Could you check a few things on this model? Use its own coordinates, in mm. A direction names the side the tool comes from. Give positions to 0.01 mm unless a question says otherwise; leave off trailing zeros. Write each loop counter-clockwise with the first axis right and the second up, starting at its lowest first coordinate (ties: lowest second). Pieces come first, ordered by that corner, then holes. Notation, with made-up numbers: (6, 13) - (18, 13) arc R21 ccw to (18, 28) - close; hole circle Ø10 at (64.5, -6.5). An arc over 180 degrees is marked (long way). Answer as CSV lines item,"result". Start each with the question number.
Q1. If I drill on line 1 along Y through (x, z) = (-18.5, 11.75); line 2 along X through (y, z) = (7.5, 13); line 3 along Y through (x, z) = (-8.5, 17.5), over which ranges is the centre line in solid material (lowest first)?
Q2. On a 3-axis mill with a long thin cutter (end or side, diameter ignored), from which of +Z, -Z, +X, -X, +Y, -Y can I reach the whole of each face in a straight line? I mean faces 4 (the face through (-10.747, -2.869, 19.184)), 5 (the face through (-8.482, -2.9, 5.6)), 6 (the face through (10, 1.232, 11)), 7 (the face through (-1.1, 3.432, 1.8)). Say none if no direction works.
Q3. We'd pull the mould along X, two halves only. Please class faces 1 (the face through (-22, -3, 8)), 2 (the face through (-19.86, 7.25, 17.38)), 3 (the face through (10, 5, 13.9)): pulls with the +X half, pulls with the -X half, needs draft (parallel to the pull), parting line crosses it, or undercut.
Q4. Imagine slicing it at D-D on z = 3.5. List the corners of the cut face in (x, y) for me.
Q5. Imagine slicing it at B-B on z = 8.75. List the corners of the cut face in (x, y) for me.
Q6. Imagine slicing it at A-A on y = 2. List the corners of the cut face in (x, z) for me, and give its area (3 significant figures).
Q7. Imagine slicing it at C-C on x = -18. List the corners of the cut face in (y, z) for me.
Q8. Will these pins go through, and if not, where does the flat tip stop? pin 1 Ø1.5 at (x, z) = (-0.5, 10) entering from +Y; pin 2 Ø8 at (y, z) = (0, 10) entering from -X; pin 3 Ø1 at (y, z) = (-2, 16.5) entering from -X; pin 4 Ø1.4 at (x, z) = (10, 12) entering from +Y.
```python
from build123d import *

# Parameters (mm, degrees)
F0_W          = 26
F0_H          = 22
F1_DEPTH      = 22
F2_R          = 9
F3_DEPTH      = 20
F4_W          = 15
F4_H          = 12.4
F5_DEPTH      = 22.001
F6_W          = 22
F6_H          = 22
F7_DEPTH      = 14
F8_W          = 18.7
F8_H          = 6
F9_DEPTH      = 12
F10_R         = 1.778
F11_DEPTH     = 40.001
F12_SIZE      = 1.5
F13_SIZE2     = 7.1236589649
F13_SIZE      = 16
F13_2_SIZE2   = 7.1236589649
F13_2_SIZE    = 16
F14_T1_DEPTH  = 27.800912408
F14_T3_DEPTH  = 27.800912408
F15_W         = 2.8
F15_H         = 5.8
F16_DEPTH     = 7
F17_W         = 22
F17_H         = 22
F18_DEPTH     = 1
F19_R         = 3.048
F20_DEPTH     = 26.5
F21_R         = 1.778
F22_DEPTH     = 6
F23_T1_DEPTH  = 2.5403411844
F23_T3_DEPTH  = 2.5403411844
F23_T5_DEPTH  = 2.5403411844
F23_T7_DEPTH  = 2.5403411844
F23_T9_DEPTH  = 32.2867319519
F23_T11_DEPTH = 32.2867319519
F23_T13_DEPTH = 30.3695452806
F24_T4_DEPTH  = 41.5282991577
F24_T10_DEPTH = 41.5282991577
F24_T16_DEPTH = 41.5282991577
F24_T22_DEPTH = 41.5282991577
F24_T28_DEPTH = 41.5282991577
F24_T34_DEPTH = 41.5282991577
F24_T40_DEPTH = 41.5282991577
F24_T46_DEPTH = 41.5282991577


# Not quite as in the source:
# - a fillet or chamfer that OpenCascade refuses, or shapes differently, is made with other operations: its cross-section is extruded or revolved along the edge and cut away or added


with BuildPart() as f1:
    # F0 (on Top) → F1 (new body)
    with BuildSketch(Plane.XY):
        with Locations((-0.9824799188, -2.7680952549)):
            Rectangle(F0_W, F0_H)
    extrude(amount=F1_DEPTH)

    # F2 (on face) → F3 (cut)
    with BuildSketch(Plane(origin=(0, 8.2319047451, 0), x_dir=(-1, 0, 0), z_dir=(0, 1, 0))):
        with Locations((0.9824799188, 11)):
            Circle(F2_R)
    extrude(amount=-F3_DEPTH, mode=Mode.SUBTRACT)

    # F4 (on face) → F5 (cut, through all)
    with BuildSketch(Plane.XY.offset(22)):
        with Locations((-0.9824799188, -2.7680952549)):
            Rectangle(F4_W, F4_H)
    extrude(amount=-F5_DEPTH, mode=Mode.SUBTRACT)

    # F6 (on face) → F7 (join)
    with BuildSketch(Plane(origin=(-13.9824799188, 0, 0), x_dir=(0, -1, 0), z_dir=(-1, 0, 0))):
        with Locations((2.7680952549, 11)):
            Rectangle(F6_W, F6_H)
    extrude(amount=F7_DEPTH)

    # F8 (on face) → F9 (cut)
    with BuildSketch(Plane(origin=(-27.9824799188, 0, 0), x_dir=(0, -1, 0), z_dir=(-1, 0, 0))):
        with Locations((2.7180952549, 11)):
            Rectangle(F8_W, F8_H)
    extrude(amount=-F9_DEPTH, mode=Mode.SUBTRACT)

    # F10 (on face) → F11 (cut, through all)
    with BuildSketch(Plane.YZ.offset(12.0175200812)):
        with Locations((-2.7180952549, 11)):
            Circle(F10_R)
    extrude(amount=-F11_DEPTH, mode=Mode.SUBTRACT)

    # F12
    f12_edges = [f1.edges().sort_by_distance(p)[0] for p in [
        (-0.98248, 3.431905, 22),
        (-0.98248, -8.968095, 22),
        (-0.98248, 3.431905, 0),
        (-0.98248, -8.968095, 0),
    ]]
    chamfer(f12_edges, length=F12_SIZE)

    # F13
    f13_edges = [f1.edges().sort_by_distance(p)[0] for p in [
        (-27.98248, -2.768095, 22),
    ]]
    f13_side = f1.faces().sort_by_distance((-10.474005, -2.768095, 22))[0]
    chamfer(f13_edges, length=F13_SIZE, length2=F13_SIZE2, reference=f13_side)

    # F13#2
    f13_2_edges = [f1.edges().sort_by_distance(p)[0] for p in [
        (-27.98248, -2.768095, 0),
    ]]
    f13_2_side = f1.faces().sort_by_distance((-10.474005, -2.768095, 0))[0]
    chamfer(f13_2_edges, length=F13_2_SIZE, length2=F13_2_SIZE2, reference=f13_2_side)

    # F14: chamfer of 2 on 4 edges, made by hand

    # F14_s2 → F14_t1 (cut)
    with BuildSketch(Plane(origin=(2.8731297183, 0, 1.2791997672), x_dir=(0, 1, 0), z_dir=(-0.9135454576, 0, -0.4067366431))):
        Polygon((8.2319047451, -22.971713726), (6.2319047451, -24.971713726), (8.2319047451, -24.971713726), align=None)
        Polygon((-11.7680952549, -24.971713726), (-13.7680952549, -22.971713726), (-13.7680952549, -24.971713726), align=None)
    extrude(amount=F14_T1_DEPTH, mode=Mode.SUBTRACT)

    # F14_s4 → F14_t3 (cut)
    with BuildSketch(Plane(origin=(-5.301463362, 0, 2.3603635629), x_dir=(0, 1, 0), z_dir=(-0.9135454576, 0, 0.4067366431))):
        Polygon((8.2319047451, 2.8737136579), (6.2319047451, 4.8737136579), (8.2319047451, 4.8737136579), align=None)
        Polygon((-11.7680952549, 4.8737136579), (-13.7680952549, 2.8737136579), (-13.7680952549, 4.8737136579), align=None)
    extrude(amount=F14_T3_DEPTH, mode=Mode.SUBTRACT)

    # F15 (on face) → F16 (cut)
    with BuildSketch(Plane(origin=(0, 8.2319047451, 0), x_dir=(-1, 0, 0), z_dir=(0, 1, 0))):
        with Locations((-10.0175200812, 11)):
            Rectangle(F15_W, F15_H)
    extrude(amount=-F16_DEPTH, mode=Mode.SUBTRACT)

    # F17 (on face) → F18 (join)
    with BuildSketch(Plane.YZ.offset(12.0175200812)):
        with Locations((-2.7680952549, 11)):
            Rectangle(F17_W, F17_H)
    extrude(amount=F18_DEPTH)

    # F19 (on face) → F20 (cut)
    with BuildSketch(Plane.YZ.offset(13.0175200812)):
        with Locations((-2.7680952549, 11)):
            Circle(F19_R)
    extrude(amount=-F20_DEPTH, mode=Mode.SUBTRACT)

    # F21 (on face) → F22 (cut)
    with BuildSketch(Plane.YZ.offset(13.0175200812)):
        with Locations((4.2319047451, 10.9924701974)):
            Circle(F21_R)
    extrude(amount=-F22_DEPTH, mode=Mode.SUBTRACT)

    # F23: chamfer of 2 on 8 edges, made by hand

    # F23_s2 → F23_t1 (cut)
    with BuildSketch(Plane(origin=(7.595205112, -7.595205112, -7.595205112), x_dir=(0.7071067812, 0.7071067812, 0), z_dir=(0.5773502692, -0.5773502692, -0.5773502692))):
        Polygon((-0.5307367951, 9.3021885081), (0.8834767672, 11.7516782509), (-1.9449503575, 11.7516782509), align=None)
    extrude(amount=F23_T1_DEPTH, mode=Mode.SUBTRACT)

    # F23_s4 → F23_t3 (cut)
    with BuildSketch(Plane(origin=(5.7498082754, 5.7498082754, -5.7498082754), x_dir=(-0.7071067812, 0.7071067812, 0), z_dir=(0.5773502692, 0.5773502692, -0.5773502692))):
        Polygon((-1.9697274939, 9.4915379396), (-3.3839410563, 7.0420481968), (-4.7981546187, 9.4915379396), align=None)
    extrude(amount=F23_T3_DEPTH, mode=Mode.SUBTRACT)

    # F23_s6 → F23_t5 (cut)
    with BuildSketch(Plane(origin=(13.0831416088, 13.0831416088, 13.0831416088), x_dir=(-0.7071067812, 0.7071067812, 0), z_dir=(0.5773502692, 0.5773502692, 0.5773502692))):
        Polygon((-1.9697274939, 8.4713868408), (-3.3839410563, 10.9208765836), (-4.7981546187, 8.4713868408), align=None)
    extrude(amount=F23_T5_DEPTH, mode=Mode.SUBTRACT)

    # F23_s8 → F23_t7 (cut)
    with BuildSketch(Plane(origin=(14.9285384454, -14.9285384454, 14.9285384454), x_dir=(0.7071067812, 0.7071067812, 0), z_dir=(0.5773502692, -0.5773502692, 0.5773502692))):
        Polygon((-0.5307367951, 8.6607362723), (0.8834767672, 6.2112465295), (-1.9449503575, 6.2112465295), align=None)
    extrude(amount=F23_T7_DEPTH, mode=Mode.SUBTRACT)

    # F23_s10 → F23_t9 (cut)
    with BuildSketch(Plane.XZ.offset(-13.375270721)):
        Polygon((11.0175200812, 0), (13.0175200812, 2), (13.0175200812, 0), align=None)
        Polygon((11.0175200812, 22), (13.0175200812, 20), (13.0175200812, 22), align=None)
    extrude(amount=F23_T9_DEPTH, mode=Mode.SUBTRACT)

    # F23_s12 → F23_t11 (cut)
    with BuildSketch(Plane.XY.offset(-5.1433659759)):
        Polygon((11.0175200812, 8.2319047451), (13.0175200812, 6.2319047451), (13.0175200812, 8.2319047451), align=None)
        Polygon((13.0175200812, -11.7680952549), (11.0175200812, -13.7680952549), (13.0175200812, -13.7680952549), align=None)
    extrude(amount=F23_T11_DEPTH, mode=Mode.SUBTRACT)

    # F23_s14 → F23_t13 (cut)
    with BuildSketch(Plane.YZ.offset(-12.2086592235)):
        Polygon((8.2319047451, 20), (6.2319047451, 22), (8.2319047451, 22), align=None)
        Polygon((-11.7680952549, 22), (-13.7680952549, 20), (-13.7680952549, 22), align=None)
        Polygon((-11.7680952549, 0), (-13.7680952549, 2), (-13.7680952549, 0), align=None)
        Polygon((8.2319047451, 2), (6.2319047451, 0), (8.2319047451, 0), align=None)
    extrude(amount=F23_T13_DEPTH, mode=Mode.SUBTRACT)

    # F24: chamfer of 5.08 on 4 edges, made by hand


with BuildPart() as f24_tool2:
    # F24_s3 → F24_t4 (new body)
    with BuildSketch(Plane.XZ.offset(23.5322448338)):
        Polygon((-8.4824799188, 16.92), (-13.5624799188, 22), (-8.4824799188, 22), align=None)
    extrude(amount=-F24_T4_DEPTH)

    split(bisect_by=Plane(origin=(0, 5.7659523726, 5.7659523726), x_dir=(1, 0, 0), z_dir=(0, 0.7071067812, 0.7071067812)), keep=Keep.TOP)

    split(bisect_by=Plane(origin=(0, -8.5340476274, 8.5340476274), x_dir=(1, 0, 0), z_dir=(0, -0.7071067812, 0.7071067812)), keep=Keep.TOP)


with BuildPart() as f1_1:
    add(f1.part)

    # F24_t1: cut F24_tool2
    add(f24_tool2.part, mode=Mode.SUBTRACT)


with BuildPart() as f24_tool8:
    # F24_s9 → F24_t10 (new body)
    with BuildSketch(Plane.XZ.offset(23.5322448338)):
        Polygon((-8.4824799188, 16.92), (-13.5624799188, 22), (-8.4824799188, 22), align=None)
    extrude(amount=-F24_T10_DEPTH)

    split(bisect_by=Plane.XZ.offset(8.9680952549), keep=Keep.BOTTOM)

    split(bisect_by=Plane.XZ.offset(-3.4319047451), keep=Keep.TOP)


with BuildPart() as f1_2:
    add(f1_1.part)

    # F24_t7: cut F24_tool8
    add(f24_tool8.part, mode=Mode.SUBTRACT)


with BuildPart() as f24_tool14:
    # F24_s15 → F24_t16 (new body)
    with BuildSketch(Plane.XZ.offset(-17.996054324)):
        Polygon((6.5175200812, 16.92), (11.5975200812, 22), (6.5175200812, 22), align=None)
    extrude(amount=F24_T16_DEPTH)

    split(bisect_by=Plane(origin=(0, 5.7659523726, 5.7659523726), x_dir=(1, 0, 0), z_dir=(0, 0.7071067812, 0.7071067812)), keep=Keep.TOP)

    split(bisect_by=Plane(origin=(0, -8.5340476274, 8.5340476274), x_dir=(1, 0, 0), z_dir=(0, -0.7071067812, 0.7071067812)), keep=Keep.TOP)


with BuildPart() as f1_3:
    add(f1_2.part)

    # F24_t13: cut F24_tool14
    add(f24_tool14.part, mode=Mode.SUBTRACT)


with BuildPart() as f24_tool20:
    # F24_s21 → F24_t22 (new body)
    with BuildSketch(Plane.XZ.offset(-17.996054324)):
        Polygon((6.5175200812, 16.92), (11.5975200812, 22), (6.5175200812, 22), align=None)
    extrude(amount=F24_T22_DEPTH)

    split(bisect_by=Plane.XZ.offset(8.9680952549), keep=Keep.BOTTOM)

    split(bisect_by=Plane.XZ.offset(-3.4319047451), keep=Keep.TOP)


with BuildPart() as f1_4:
    add(f1_3.part)

    # F24_t19: cut F24_tool20
    add(f24_tool20.part, mode=Mode.SUBTRACT)


with BuildPart() as f24_tool26:
    # F24_s27 → F24_t28 (new body)
    with BuildSketch(Plane.XZ.offset(23.5322448338)):
        Polygon((11.5975200812, 0), (6.5175200812, 5.08), (6.5175200812, 0), align=None)
    extrude(amount=-F24_T28_DEPTH)

    split(bisect_by=Plane.XZ.offset(8.9680952549), keep=Keep.BOTTOM)

    split(bisect_by=Plane(origin=(0, 2.4659523726, 2.4659523726), x_dir=(1, 0, 0), z_dir=(0, -0.7071067812, -0.7071067812)), keep=Keep.TOP)


with BuildPart() as f1_5:
    add(f1_4.part)

    # F24_t25: cut F24_tool26
    add(f24_tool26.part, mode=Mode.SUBTRACT)


with BuildPart() as f24_tool32:
    # F24_s33 → F24_t34 (new body)
    with BuildSketch(Plane.XZ.offset(23.5322448338)):
        Polygon((11.5975200812, 0), (6.5175200812, 5.08), (6.5175200812, 0), align=None)
    extrude(amount=-F24_T34_DEPTH)

    split(bisect_by=Plane.XZ.offset(-3.4319047451), keep=Keep.TOP)

    split(bisect_by=Plane(origin=(0, -5.2340476274, 5.2340476274), x_dir=(1, 0, 0), z_dir=(0, 0.7071067812, -0.7071067812)), keep=Keep.TOP)


with BuildPart() as f1_6:
    add(f1_5.part)

    # F24_t31: cut F24_tool32
    add(f24_tool32.part, mode=Mode.SUBTRACT)


with BuildPart() as f24_tool38:
    # F24_s39 → F24_t40 (new body)
    with BuildSketch(Plane.XZ.offset(-17.996054324)):
        Polygon((-13.5624799188, 0), (-8.4824799188, 5.08), (-8.4824799188, 0), align=None)
    extrude(amount=F24_T40_DEPTH)

    split(bisect_by=Plane.XZ.offset(-3.4319047451), keep=Keep.TOP)

    split(bisect_by=Plane(origin=(0, -5.2340476274, 5.2340476274), x_dir=(1, 0, 0), z_dir=(0, 0.7071067812, -0.7071067812)), keep=Keep.TOP)


with BuildPart() as f1_7:
    add(f1_6.part)

    # F24_t37: cut F24_tool38
    add(f24_tool38.part, mode=Mode.SUBTRACT)


with BuildPart() as f24_tool44:
    # F24_s45 → F24_t46 (new body)
    with BuildSketch(Plane.XZ.offset(-17.996054324)):
        Polygon((-13.5624799188, 0), (-8.4824799188, 5.08), (-8.4824799188, 0), align=None)
    extrude(amount=F24_T46_DEPTH)

    split(bisect_by=Plane.XZ.offset(8.9680952549), keep=Keep.BOTTOM)

    split(bisect_by=Plane(origin=(0, 2.4659523726, 2.4659523726), x_dir=(1, 0, 0), z_dir=(0, -0.7071067812, -0.7071067812)), keep=Keep.TOP)


with BuildPart() as f1_8:
    add(f1_7.part)

    # F24_t43: cut F24_tool44
    add(f24_tool44.part, mode=Mode.SUBTRACT)


solid = f1_8.part
```
Conclusion:
1,line 1,"-13.77 to -12.07, 6.63 to 8.23"
1,line 2,"-27.98 to -9.76, 7.79 to 8.62, 11.42 to 11.75"
1,line 3,"-13.77 to -8.97, 3.43 to 8.23"
2,face 4,"+Z"
2,face 5,"+Z, -Z"
2,face 6,"+Y"
2,face 7,"-Z"
3,face 1,"needs draft"
3,face 2,"pulls with the -X half"
3,face 3,"undercut"
4,outline,"(-19.84, -11.77) - (-14.93, -13.77) - (11.02, -13.77) - (13.02, -11.77) - (13.02, 6.23) - (11.02, 8.23) - (3.99, 8.23) - (3.99, 3.43) - (8.1, 3.43) - (8.1, -8.97) - (3.99, -8.97) - (3.99, -11.77) - (-5.96, -11.77) - (-5.96, -8.97) - (-10.06, -8.97) - (-10.06, 3.43) - (-5.96, 3.43) - (-5.96, 8.23) - (-14.93, 8.23) - (-19.84, 6.23) - close"
5,outline,"(-27.98, -13.25) - (-26.72, -13.77) - (11.02, -13.77) - (13.02, -11.77) - (13.02, -4.82) - (7.73, -4.82) - (7.73, -11.77) - (-9.7, -11.77) - (-9.7, -4.82) - (-13.48, -4.82) - (-13.48, -0.71) - (-9.7, -0.71) - (-9.7, 8.23) - (-26.72, 8.23) - (-27.98, 7.72) - (-27.98, 6.63) - (-15.98, 6.63) - (-15.98, -12.07) - (-27.98, -12.07) - close; (7.73, -0.71) - (13.02, -0.71) - (13.02, 6.23) - (11.42, 7.83) - (11.42, 1.23) - (8.62, 1.23) - (8.62, 8.23) - (7.73, 8.23) - close"
6,outline,"(-27.98, 7.12) - (-13.08, 0.49) - (-8.48, 5.08) - (-8.48, 6.03) arc R9 cw to (-8.48, 15.97) - (-8.48, 16.92) - (-13.08, 21.51) - (-27.98, 14.88) - (-27.98, 14) - (-15.98, 14) - (-15.98, 8) - (-27.98, 8) - close; (6.52, 5.08) - (11.31, 0.29) - (13.02, 2) - (13.02, 20) - (11.31, 21.71) - (6.52, 16.92) - (6.52, 15.97) arc R9 cw to (6.52, 6.03) - close; hole (8.62, 8.1) - (11.42, 8.1) - (11.42, 13.9) - (8.62, 13.9) - close"
6,area,"295 mm^2"
7,outline,"(-13.77, 4.87) - (-11.77, 2.68) - (6.23, 2.68) - (8.23, 4.87) - (8.23, 17.13) - (6.23, 19.32) - (-11.77, 19.32) - (-13.77, 17.13) - close; hole (-12.07, 8) - (6.63, 8) - (6.63, 14) - (-12.07, 14) - close"
8,pin 1,"y = -11.77"
8,pin 2,"x = -27.98"
8,pin 3,"x = -25.46"
8,pin 4,"y = 1.23"
